Verification items for the finished model (mm, model axes). A direction names the side the tool comes from. Give positions to 0.01 mm unless a question says otherwise; leave off trailing zeros. Order: outer loops, then holes, each group sorted by start corner. A loop starts at its lowest first (then second) coordinate and runs counter-clockwise, first axis right, second up.
Autodesk Inventor part; units mm, degrees
ref_plane "YZ Plane" through (0, 0, 0) normal (1, 0, 0) x (0, 1, 0)
ref_plane "XZ Plane" through (0, 0, 0) normal (0, 1, 0) x (-1, 0, 0)
ref_plane "XY Plane" through (0, 0, 0) normal (0, 0, 1) x (1, 0, 0)
sketch "Sketch1" plane through (0, 0, 0) normal (0, 1, 0) x (-1, 0, 0)
  line L0 (-20, 20) -> (20, 20)
  line L1 (20, 20) -> (20, -20)
  line L2 (20, -20) -> (-20, -20)
  line L3 (-20, -20) -> (-20, 20)
  line L4 (-20, 20) -> (20, -20) construction
  line L5 (20, 20) -> (-20, -20) construction
  circle A0 centre (0, 0) radius 4
  circle A1 centre (0, 8.5) radius 1.75
  circle A2 centre (0, -8.5) radius 1.75
  point P0 (0, 0)
  point P1 (0, 0)
  dimension "d0" = 40
  dimension "d1" = 40
  dimension "d2" = 8
  dimension "d3" = 3.5
  dimension "d4" = 3.5
  dimension "d5" = 8.5
  dimension "d6" = 8.5
extrude "Extrusion1" add sketch "Sketch1" along normal blind 3
chamfer "Chamfer1" distance 2 angle 45 2 edges at (1.75, 3, -8.5) (1.75, 3, 8.5)
fillet "Fillet1" radius 8 4 edges at (-20, 1.5, -20) (-20, 1.5, 20) (20, 1.5, -20) (20, 1.5, 20)
sketch "Sketch3" plane through (0, 3, 0) normal (0, 1, 0) x (1, 0, 0)
  circle A0 centre (-15, -15) radius 1.75
  circle A1 centre (-15, 15) radius 1.75
  circle A2 centre (15, 15) radius 1.75
  circle A3 centre (15, -15) radius 1.75
  point P0 (0, 0)
  dimension "d13" = 3.5
  dimension "d14" = 15
  dimension "d15" = 15
  dimension "d16" = 15
  dimension "d17" = 15
extrude "Extrusion2" cut sketch "Sketch3" against normal through all
sketch "Sketch4" plane through (0, 0, 0) normal (0, -1, 0) x (1, 0, 0)
  circle A0 centre (0, 0) radius 12.75
  circle A1 centre (-15, 15) radius 1.75
  circle A2 centre (15, -15) radius 1.75
  circle A3 centre (15, 15) radius 1.75
  circle A4 centre (-15, -15) radius 1.75
  arc A5 (20, 12) -> (12, 20) centre (12, 12) ccw
  line L0 (-12, 20) -> (12, 20)
  arc A6 (-12, 20) -> (-20, 12) centre (-12, 12) ccw
  line L1 (-20, -12) -> (-20, 12)
  arc A7 (-20, -12) -> (-12, -20) centre (-12, -12) ccw
  line L2 (12, -20) -> (-12, -20)
  arc A8 (12, -20) -> (20, -12) centre (12, -12) ccw
  line L3 (20, 12) -> (20, -12)
  circle A9 centre (0, -8.5) radius 1.75
  circle A10 centre (0, 8.5) radius 1.75
  circle A11 centre (0, 0) radius 4
  dimension "d22" = 25.5
extrude "Extrusion3" add sketch "Sketch4" along normal blind 20 contours L3 A8 L2 A7 L1 A6 L0 A5
fillet "Fillet2" radius 2 1 edges at (-12.75, -20, 0)
properties part number "soportemotor"
(1) Scan lines: line 1 (Z direction, x = 0, y = -9.25); line 2 (Z direction, x = 15, y = -10). Record each from-to range of solid material in increasing order.
Solved:
line 1: z = -20 to -12.75, 12.75 to 20
line 2: z = -19.42 to -16.75, -13.25 to 13.25, 16.75 to 19.42
(2) Section check C-C, the plane y = -12.75. Enter the section's corners in (x, z).
Solved:
outline: (-20, -12) arc R8 ccw to (-12, -20) - (12, -20) arc R8 ccw to (20, -12) - (20, 12) arc R8 ccw to (12, 20) - (-12, 20) arc R8 ccw to (-20, 12) - close; hole circle Ø3.5 at (-15, -15); hole circle Ø3.5 at (-15, 15); hole circle Ø25.5 at (0, 0); hole circle Ø3.5 at (15, -15); hole circle Ø3.5 at (15, 15)
(3) Section check A-A, the plane x = 0. Enter the section's corners in (y, z).
Solved:
outline: (-20, -20) - (3, -20) - (3, -12.25) - (1, -10.25) - (0, -10.25) - (0, -12.75) - (-18, -12.75) arc R2 ccw to (-20, -14.75) - close; (-20, 14.75) arc R2 ccw to (-18, 12.75) - (0, 12.75) - (0, 10.25) - (1, 10.25) - (3, 12.25) - (3, 20) - (-20, 20) - close; (0, -6.75) - (1, -6.75) - (3, -4.75) - (3, -4) - (0, -4) - close; (0, 4) - (3, 4) - (3, 4.75) - (1, 6.75) - (0, 6.75) - close
(4) Section check B-B, the plane z = 0. Enter the section's corners in (x, y), then the cut area to 3 significant figures.
Solved:
outline: (-20, -20) - (-14.75, -20) arc R2 ccw to (-12.75, -18) - (-12.75, 0) - (-4, 0) - (-4, 3) - (-20, 3) - close; (4, 0) - (12.75, 0) - (12.75, -18) arc R2 ccw to (14.75, -20) - (20, -20) - (20, 3) - (4, 3) - close
area: 384 mm2
(5) Release check for a two-part mould opening along X. For faces 1 (the cylindrical face through (-17.719, -8.339, 17.594)), 2 (the cylindrical face through (-2.764, -8.874, 12.447)), 3 (the flat face through (-4.2, 3, 0.3)), 4 (the cylindrical face through (14.772, -8.339, 13.265)) record: pulls with the +X half, pulls with the -X half, needs draft (parallel to the pull), parting line crosses it, or undercut.
Solved:
face 1: pulls with the -X half
face 2: undercut
face 3: needs draft
face 4: undercut
(6) Go/stop test with a flat-tipped pin: pin 1 (5.5 mm diameter, centred on x = 0, z = -8.5, fed in from -Y). Record where the tip stops, or that it passes through.
Solved:
pin 1: stops at y = 0
(7) Set-up check for faces 5 (the cylindrical face through (-0.9, 0.5, 7)), 6 (the flat face through (-3, 0, 3)): record each of +Z, -Z, +X, -X, +Y, -Y from which the full face is reachable in a straight line by a thin tool's end or side.
Solved:
face 5: +Y, -Y
face 6: -Y
